Build history of the part. All positions in model axes, mm. A direction names the side the tool comes from. Give positions to 0.01 mm unless a question says otherwise; leave off trailing zeros. Order: outer loops, then holes, each group sorted by start corner. A loop starts at its lowest first (then second) coordinate and runs counter-clockwise, first axis right, second up. Notation, with made-up numbers: M 7.5,17.25 L 27.5,17.25 A15 ccw 27.5,42.25 Z; hole C 31.5,6 d9. An arc over 180 degrees is marked long. One line per item, written item: value.
from build123d import *

# Parameters (mm, degrees)
SKETCH3_W           = 24
SKETCH3_H           = 24
BOSS_EXTRUDE1_DEPTH = 8
FILLET1_R           = 5


with BuildPart() as part:
    # Sketch1 → Revolve1 (revolve)
    with BuildSketch(Plane.XY, mode=Mode.PRIVATE) as revolve1_sk:
        Polygon((0, 56), (-12, 56), (-12, 48), (-6, 48), (-6, -48), (0, -48), align=None)
    revolve(revolve1_sk.sketch.rotate(Axis((0, -48, 0), (0, 1, 0)), 180), axis=Axis((0, -48, 0), (0, 1, 0)))

    # Sketch3 → Boss-Extrude1 (add)
    with BuildSketch(Plane.XZ.offset(-48)):
        Rectangle(SKETCH3_W, SKETCH3_H)
    extrude(amount=-BOSS_EXTRUDE1_DEPTH)

    # Fillet1
    fillet1_edges = [part.edges().sort_by_distance(p)[0] for p in [
        (-12, 56, 0),
        (0, 56, 12),
        (12, 56, 0),
        (0, 56, -12),
    ]]
    fillet(fillet1_edges, radius=FILLET1_R)


solid = part.part
1) Pin check, flat tips, straight feed: pin 1 (8 mm diameter, centred on y = 38, z = 1.5, fed in from -X); pin 2 (1 mm diameter, centred on x = -2, y = -29.5, fed in from +Z). Stop position of each tip, or through.
Check values:
pin 1: x = -6
pin 2: z = 5.81
2) Saw through at B-B, the plane z = 0. Write the cut outline in (x, y), then the cut area to 3 significant figures.
Check values:
outline: M -12,48 L -6,48 L -6,-48 L 6,-48 L 6,48 L 12,48 L 12,51 A5 ccw 7,56 L -7,56 A5 ccw -12,51 Z
area: 1,330 mm^2
3) Drill centre lines: probe 1 along Y at (x, z) = (6.75, 3.25); probe 2 along Z at (x, y) = (0.5, 47); probe 3 along Y at (x, z) = (-10.75, 10). Where is each one in solid material? Low to high. Write a range as from..to.
Check values:
probe 1: 48..56
probe 2: -5.98..5.98
probe 3: 48..54.31
4) Saw through at A-A, the plane x = 0. Write the cut outline in (y, z).
Check values:
outline: M -48,-6 L 48,-6 L 48,-12 L 51,-12 A5 ccw 56,-7 L 56,7 A5 ccw 51,12 L 48,12 L 48,6 L -48,6 Z
5) Saw through at D-D, the plane z = 10.25. Write the cut outline in (x, y), then the cut area to 3 significant figures.
Check values:
outline: M -12,48 L 12,48 L 12,51 A5 ccw 10.25,54.8 L -10.25,54.8 A5 ccw -12,51 Z
area: 159 mm^2
6) Saw through at C-C, the plane y = 40. Write the cut outline in (x, z).
Check values:
outline: C 0,0 d12
7) Tool access for faces 1 (the face through (-6, 48, 3)), 2 (the face through (0, 56, 0)): list every direction of +Z, -Z, +X, -X, +Y, -Y with a clear straight run to the whole face (end or side of a thin tool).
Check values:
face 1: -Y
face 2: +Z, -Z, +X, -X, +Y
